For this review, take the finished solid that the model builds, in its own axes (mm). Coordinates: 2 decimals unless noted, no trailing zeros. Write each loop counter-clockwise with the first axis right and the second up, starting at its lowest first coordinate (ties: lowest second). Pieces come first, ordered by that corner, then holes.
1) We need section C-C on y = 34.5. Write out the cut boundary in (x, z) (3 decimals), then the cut area to 3 significant figures.
2) To check wall thickness, follow line 1 along Y through (x, z) = (13.5, -7); line 2 along Z through (x, y) = (1.25, 30); line 3 along Z through (x, y) = (21.75, -9). State the ranges of each line that lie inside material, in increasing order.
3) Insertion check: P1, Ø6, axis at x = 14.5, z = 28.5, coming from the +Y side. The pin has a flat end and moves straight along its axis. Give the tip position at first contact, or say it passes through.
4) We need section A-A on x = 20. Write out the cut boundary in (y, z), then the cut area to 3 significant figures.
5) We need section B-B on z = -2.5. Write out the cut boundary in (x, y), then the cut area to 3 significant figures.
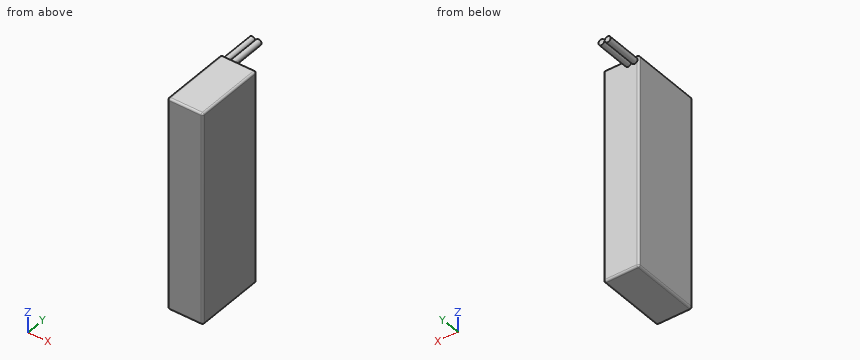
from build123d import *

# Parameters (mm, degrees)
SKETCH1_W           = 137.16
SKETCH1_H           = 45.72
BOSS_EXTRUDE1_DEPTH = 22.86
FILLET1_R           = 1.27
SKETCH2_R           = 1.905
BOSS_EXTRUDE2_DEPTH = 22.86


with BuildPart() as part:
    # Sketch1 → Boss-Extrude1 (new body)
    with BuildSketch(Plane(origin=(0, 0, 0), x_dir=(0, 0, -1), z_dir=(1, 0, 0))):
        Rectangle(SKETCH1_W, SKETCH1_H)
    extrude(amount=BOSS_EXTRUDE1_DEPTH)

    # Fillet1
    fillet1_edges = [part.edges().sort_by_distance(p)[0] for p in [
        (22.86, 0, 68.58),
        (22.86, -22.86, 0),
        (22.86, 0, -68.58),
        (0, -22.86, 0),
        (0, 0, 68.58),
        (0, 22.86, 0),
        (0, 0, -68.58),
        (22.86, 22.86, 0),
        (11.43, -22.86, -68.58),
        (11.43, -22.86, 68.58),
        (11.43, 22.86, 68.58),
        (11.43, 22.86, -68.58),
    ]]
    fillet(fillet1_edges, radius=FILLET1_R)

    # Sketch2 → Boss-Extrude2 (add)
    with BuildSketch(Plane(origin=(0, 22.86, 0), x_dir=(1, 0, 0), z_dir=(0, 1, 0))):
        with Locations((2.722644531, -65.585417965)):
            Circle(SKETCH2_R)
        with Locations((6.786644531, -65.585417965)):
            Circle(SKETCH2_R)
    extrude(amount=BOSS_EXTRUDE2_DEPTH)


solid = part.part
Result:
1. outline: circle Ø3.81 at (2.723, 65.585); circle Ø3.81 at (6.787, 65.585)
1. area: 22.8 mm2
2. line 1: y = -22.86 to 22.86
2. line 2: z = 64.38 to 66.79
2. line 3: z = -68.57 to 68.57
3. P1: stops at y = 22.86
4. outline: (-22.86, -67.31) arc R1.27 ccw to (-21.59, -68.58) - (21.59, -68.58) arc R1.27 ccw to (22.86, -67.31) - (22.86, 67.31) arc R1.27 ccw to (21.59, 68.58) - (-21.59, 68.58) arc R1.27 ccw to (-22.86, 67.31) - close
4. area: 6,270 mm2
5. outline: (0, -21.59) arc R1.27 ccw to (1.27, -22.86) - (21.59, -22.86) arc R1.27 ccw to (22.86, -21.59) - (22.86, 21.59) arc R1.27 ccw to (21.59, 22.86) - (1.27, 22.86) arc R1.27 ccw to (0, 21.59) - close
5. area: 1,040 mm2
